Verification items for the finished model (mm, model axes). A direction names the side the tool comes from. Round coordinates to 2 decimals unless told otherwise and drop trailing zeros. Write each loop counter-clockwise with the first axis right and the second up, starting at its lowest first coordinate (ties: lowest second). Pieces come first, ordered by that corner, then holes. Notation, with made-up numbers: (23, -39.75) -> (71, -39.75) arc R18 ccw to (71, -9.75) -> close; hole circle Ø7 at (15, 80). An arc over 180 degrees is marked (long way). Use CSV: the item, a comma, the result in double quotes.
```python
from build123d import *

# Parameters (mm, degrees)
SKETCH1_W           = 78
SKETCH1_H           = 25
BOSS_EXTRUDE1_DEPTH = 4
SKETCH2_R           = 2.5
SKETCH2_W           = 46
SKETCH2_H           = 2.5
BOSS_EXTRUDE2_DEPTH = 7
SKETCH3_W           = 5.5
SKETCH3_H           = 10
BOSS_EXTRUDE3_DEPTH = 6.5
SKETCH4_R           = 2
CUT_EXTRUDE1_DEPTH  = 10


with BuildPart() as part:
    # Sketch1 → Boss-Extrude1 (new body)
    with BuildSketch(Plane(origin=(0, 0, 0), x_dir=(1, 0, 0), z_dir=(0, 1, 0))):
        Rectangle(SKETCH1_W, SKETCH1_H)
    extrude(amount=BOSS_EXTRUDE1_DEPTH)

    # Sketch2 → Boss-Extrude2 (add)
    with BuildSketch(Plane(origin=(0, 4, 0), x_dir=(1, 0, 0), z_dir=(0, 1, 0))):
        with Locations(Location((28, -7.5, 0), (0, 0, 90))):
            Circle(SKETCH2_R)
        with Locations((0, -9.75)):
            Rectangle(SKETCH2_W, SKETCH2_H)
    extrude(amount=BOSS_EXTRUDE2_DEPTH)

    # Sketch3 → Boss-Extrude3 (add)
    with BuildSketch(Plane.XZ):
        with Locations((-35.25, -7.5)):
            Rectangle(SKETCH3_W, SKETCH3_H)
        with Locations((-25.178571429, -7.5)):
            Rectangle(SKETCH3_W, SKETCH3_H)
        with Locations((-15.107142857, -7.5)):
            Rectangle(SKETCH3_W, SKETCH3_H)
        with Locations((-5.035714286, -7.5)):
            Rectangle(SKETCH3_W, SKETCH3_H)
        with Locations((5.035714286, -7.5)):
            Rectangle(SKETCH3_W, SKETCH3_H)
        with Locations((15.107142857, -7.5)):
            Rectangle(SKETCH3_W, SKETCH3_H)
        with Locations((25.178571429, -7.5)):
            Rectangle(SKETCH3_W, SKETCH3_H)
        with Locations((35.25, -7.5)):
            Rectangle(SKETCH3_W, SKETCH3_H)
    extrude(amount=BOSS_EXTRUDE3_DEPTH)

    # Sketch4 → Cut-Extrude1 (cut)
    with BuildSketch(Plane(origin=(0, 4, 0), x_dir=(1, 0, 0), z_dir=(0, 1, 0))):
        with Locations(Location((-36.5, -2, 0), (0, 0, 270))):
            Circle(SKETCH4_R)
        with Locations(Location((36.5, -2, 0), (0, 0, 90))):
            Circle(SKETCH4_R)
    extrude(amount=-CUT_EXTRUDE1_DEPTH, mode=Mode.SUBTRACT)


solid = part.part
```
Q1. Section check C-C (x = -36.5). Record the cut outline in (y, z), plus the area to 3 significant figures.
Filled in:
outline,"(-6.5, -12.5) -> (4, -12.5) -> (4, 0) -> (0, 0) -> (0, -2.5) -> (-6.5, -2.5) -> close; (0, 4) -> (4, 4) -> (4, 12.5) -> (0, 12.5) -> close"
area,"149 mm²"
Q2. Section check D-D (y = 9). Record the cut outline in (x, z).
Filled in:
outline,"(-23, 8.5) -> (23, 8.5) -> (23, 11) -> (-23, 11) -> close; circle Ø5 at (28, 7.5)"
Q3. Section check A-A (y = -4.5). State how many separate pieces and enclosed holes the cut face has, plus the area to 3 significant figures.
Filled in:
separate pieces,"8"
enclosed holes,"0"
area,"440 mm²"
Q4. Go/stop test with flat-tipped pins: P1, Ø2, axis at x = -0.5, y = 8, coming from the -Z side; P2, Ø7, axis at y = -4, z = -8.5, coming from the +X side; P3, Ø6.5, axis at x = -36.5, z = 2, coming from the -Y side. Record where each tip stops, or that it passes through.
Filled in:
P1,"z = 8.5"
P2,"x = 38"
P3,"y = 0"
Q5. Section check B-B (z = 2). Record the cut outline in (x, y).
Filled in:
outline,"(-39, 0) -> (-38.5, 0) -> (-38.5, 4) -> (-39, 4) -> close; (-34.5, 0) -> (34.5, 0) -> (34.5, 4) -> (-34.5, 4) -> close; (38.5, 0) -> (39, 0) -> (39, 4) -> (38.5, 4) -> close"
Q6. Access from +Z, -Z, +X, -X, +Y, -Y to the whole of each face (thin tool, end or side, straight path). Record for faces 5 (the flat face through (0, 7, 11)), 6 (the flat face through (17.857, -3, -8)), 7 (the flat face through (-15, -3, -2.5)), 8 (the flat face through (38, -3, -8)).
Filled in:
face 5,"+Z, +X, -X, +Y"
face 6,"+Z, -Z, -Y"
face 7,"+Z, +X, -X, -Y"
face 8,"+Z, -Z, +X, -Y"
Q7. Mould release check, pull along Z, two halves, no side actions. Record for faces 1 (the cylindrical face through (-38.452, 2.028, 1.566)), 2 (the cylindrical face through (25.52, 7.45, 7.83)), 3 (the flat face through (-5, -3, -2.5)), 4 (the flat face through (-12.357, -3, -8)): released by +Z, released by -Z, zero draft, split by the parting line, or undercut.
Filled in:
face 1,"undercut"
face 2,"split by the parting line"
face 3,"released by +Z"
face 4,"zero draft"
Q8. Material ranges on L1, parallel to X at y = 3.05, z = 2; L2, parallel to Z at x = 36.5, y = 2.45; L3, parallel to Y at x = 16, z = -2.25, recorded low to high.
Filled in:
L1,"-39 to -38.5, -34.5 to 34.5, 38.5 to 39"
L2,"-12.5 to 0, 4 to 12.5"
L3,"0 to 4"
